Design review of the part built by this model. Coordinates are the model's own, in mm. Face numbers are marked on the shaded views. Coordinates: 2 decimals unless noted, no trailing zeros. Write each loop counter-clockwise with the first axis right and the second up, starting at its lowest first coordinate (ties: lowest second). Pieces come first, ordered by that corner, then holes. Notation, with made-up numbers: (-6, -6.5) -> (20, -6.5) arc R7 cw to (20, 5.5) -> close; hole circle Ø5 at (69.5, 10.25). An arc over 180 degrees is marked (long way). One line per question, with ' | ' between items. Start each with the question number.
Q1. Add section A-A on z = 4.5. State the section outline as (x, y) points.
Q2. For P1, Ø1, axis at x = -3, y = 0.5, coming from the -Z side; P2, Ø2, axis at x = 0, y = 0, coming from the -Z side, all flat-tipped, find the tip position at first contact; note any pin that passes through.
Q3. Wall thickness on probe 1 along X at (y, z) = (0, 1.3); probe 2 along Y at (x, z) = (0, 2.3); probe 3 along X at (y, z) = (1, 6.25): over which ranges is each line inside the solid? List them lowest first.
Q4. Draft analysis for pull direction Y (two halves, no side actions). For the marked faces 1, 2 and 3, state which applies: pulls with the +Y half, pulls with the -Y half, needs draft (parallel to the pull), parting line crosses it, or undercut.
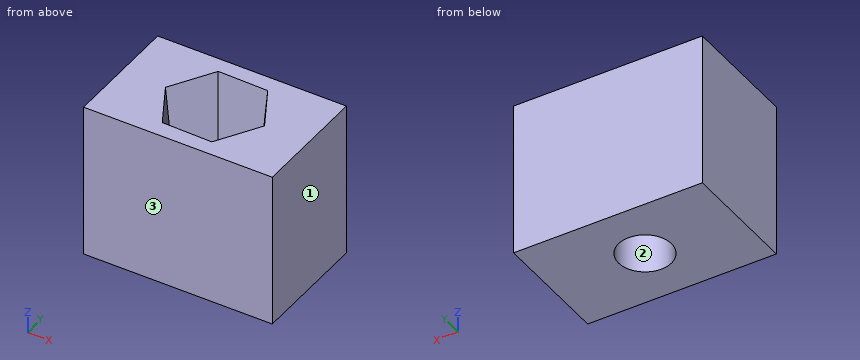
from build123d import *

# Parameters (mm, degrees)
ESQUISSE1_W             = 12.149550462
ESQUISSE1_H             = 7.67378493
ESQUISSE1_R             = 1.7
BOSS_EXTRU_1_DEPTH      = 10
ENL_V_MAT_EXTRU_1_DEPTH = 5
ENL_V_MAT_EXTRU_1_TAPER = 5


with BuildPart() as part:
    # Esquisse1 → Boss.-Extru.1 (new body)
    with BuildSketch(Plane.XY):
        Rectangle(ESQUISSE1_W, ESQUISSE1_H)
        Circle(ESQUISSE1_R, mode=Mode.SUBTRACT)
    extrude(amount=BOSS_EXTRU_1_DEPTH)

    # Esquisse2 → Enlèv. mat.-Extru.1 (cut)
    with BuildSketch(Plane.XY.offset(10)):
        Polygon((1.675518047, 2.765135188), (-1.556918294, 2.833608787), (-3.232436341, 0.068473599), (-1.675518047, -2.765135188), (1.556918294, -2.833608787), (3.232436341, -0.068473599), align=None)
    extrude(amount=-ENL_V_MAT_EXTRU_1_DEPTH, taper=ENL_V_MAT_EXTRU_1_TAPER, mode=Mode.SUBTRACT)


solid = part.part
Output values:
1) outline: (-6.07, -3.84) -> (6.07, -3.84) -> (6.07, 3.84) -> (-6.07, 3.84) -> close; hole circle Ø3.4 at (0, 0)
2) P1: stops at z = 0 | P2: passes through
3) probe 1: x = -6.07 to -1.7, 1.7 to 6.07 | probe 2: y = -3.84 to -1.7, 1.7 to 3.84 | probe 3: x = -6.07 to -2.28, 2.27 to 6.07
4) face 1: needs draft | face 2: undercut | face 3: pulls with the -Y half
